For this review, take the finished solid that the model builds, in its own axes (mm). A direction names the side the tool comes from. Round coordinates to 2 decimals unless told otherwise and drop trailing zeros. Write each loop counter-clockwise with the first axis right and the second up, starting at its lowest first coordinate (ties: lowest second). Pieces come first, ordered by that corner, then holes.
from build123d import *

# Parameters (mm, degrees)
SKETCH_1_R      = 12
SKETCH_1_R_2    = 2
EXTRUDE_1_DEPTH = 3
SKETCH_1_3_R    = 2.25
EXTRUDE_2_DEPTH = 5
EXTRUDE_START   = 3
SKETCH_1_4_R    = 6
SKETCH_1_4_R_2  = 2
EXTRUDE_3_DEPTH = 3
EXTRUDE_START_2 = 6
SKETCH_1_5_R    = 6
EXTRUDE_5_DEPTH = 1
SKETCH_2_R      = 3.5
EXTRUDE_4_DEPTH = 8


with BuildPart() as part:
    # 草图1 → 凸台-拉伸1 (new body)
    with BuildSketch(Plane.XY):
        Circle(SKETCH_1_R)
        Circle(SKETCH_1_R_2, mode=Mode.SUBTRACT)
    extrude(amount=EXTRUDE_1_DEPTH)

    # 草图1<3> → 凸台-拉伸2 (add)
    with BuildSketch(Plane.XY):
        with Locations((0, 8.4)):
            Circle(SKETCH_1_3_R)
        with Locations((7.274613392, -4.2)):
            Circle(SKETCH_1_3_R)
        with Locations((-7.274613392, -4.2)):
            Circle(SKETCH_1_3_R)
    extrude(amount=-EXTRUDE_2_DEPTH)

    # 草图1<4> → 凸台-拉伸3 (add)
    with BuildSketch(Plane.XY.offset(EXTRUDE_START)):
        Circle(SKETCH_1_4_R)
        Circle(SKETCH_1_4_R_2, mode=Mode.SUBTRACT)
    extrude(amount=EXTRUDE_3_DEPTH)

    # 草图1<5> → 凸台-拉伸5 (add)
    with BuildSketch(Plane.XY.offset(EXTRUDE_START_2)):
        Circle(SKETCH_1_5_R)
    extrude(amount=EXTRUDE_5_DEPTH)

    # 草图2 → 凸台-拉伸4 (add)
    with BuildSketch(Plane.XY.offset(7)):
        Circle(SKETCH_2_R)
        Polygon((-1.204280479, -1.204280479), (-2.304280479, -1.204280479), (-2.304280479, 1.204280479), (-1.204280479, 1.204280479), (-1.204280479, 2.304280479), (1.204280479, 2.304280479), (1.204280479, 1.204280479), (2.304280479, 1.204280479), (2.304280479, -1.204280479), (1.204280479, -1.204280479), (1.204280479, -2.304280479), (-1.204280479, -2.304280479), align=None, mode=Mode.SUBTRACT)
    extrude(amount=EXTRUDE_4_DEPTH)


solid = part.part
(1) For pin 1 Ø0.6 at (x, z) = (2, 11) entering from +Y; pin 2 Ø2.5 at (y, z) = (0, 12) entering from +X; pin 3 Ø1.9 at (x, z) = (0, 11) entering from +Y, all flat-tipped, find the tip position at first contact; note any pin that passes through.
Geometry check:
pin 1: stops at y = 3.06
pin 2: stops at x = 3.5
pin 3: stops at y = 3.5
(2) For faces 4 (the face through (0, -2, 3)), 5 (the face through (0, 2.304, 11)), 6 (the face through (-7, -4, -5)), list the 3-axis set-ups (+Z, -Z, +X, -X, +Y, -Y) from which the entire face can be reached by the end or side of a thin tool; tool diameter is ignored.
Geometry check:
face 4: -Z
face 5: +Z
face 6: -Z, +X, -X, +Y, -Y
(3) For line 1 along Y through (x, z) = (0, 1.3); line 2 along Z through (x, y) = (6.75, -0.75); line 3 along Z through (x, y) = (-0.75, 1.5), list the stretches that pass through material, from the lowest coordinate up.
Geometry check:
line 1: y = -12 to -2, 2 to 12
line 2: z = 0 to 3
line 3: z = 6 to 7
(4) We need section B-B, the plane x = 0. Give the boundary of the cut face in (y, z), and give its area (3 significant figures).
Geometry check:
outline: (-12, 0) - (-2, 0) - (-2, 6) - (2, 6) - (2, 0) - (6.15, 0) - (6.15, -5) - (10.65, -5) - (10.65, 0) - (12, 0) - (12, 3) - (6, 3) - (6, 7) - (3.5, 7) - (3.5, 15) - (2.3, 15) - (2.3, 7) - (-2.3, 7) - (-2.3, 15) - (-3.5, 15) - (-3.5, 7) - (-6, 7) - (-6, 3) - (-12, 3) - close
area: 138 mm2
(5) We need section A-A, the plane z = 9.75. Give the boundary of the cut face in (x, y).
Geometry check:
outline: circle Ø7 at (0, 0); hole (-2.3, -1.2) - (-1.2, -1.2) - (-1.2, -2.3) - (1.2, -2.3) - (1.2, -1.2) - (2.3, -1.2) - (2.3, 1.2) - (1.2, 1.2) - (1.2, 2.3) - (-1.2, 2.3) - (-1.2, 1.2) - (-2.3, 1.2) - close
(6) We need section D-D, the plane z = -3.5. Give the boundary of the cut face in (x, y), and give its area (3 significant figures).
Geometry check:
outline: circle Ø4.5 at (-7.27, -4.2); circle Ø4.5 at (0, 8.4); circle Ø4.5 at (7.27, -4.2)
area: 47.7 mm2
(7) Mouldability with a two-part tool opening along X and no side actions: class faces 1 (the face through (3, -3, 7)), 2 (the face through (-11.99, 0.53, 1.48)), 3 (the face through (1.204, 2, 11)) as pulls with the +X half, pulls with the -X half, needs draft (parallel to the pull), parting line crosses it, or undercut.
Geometry check:
face 1: needs draft
face 2: parting line crosses it
face 3: undercut
(8) We need section C-C, the plane y = 0. Give the boundary of the cut face in (x, z), and give its area (3 significant figures).
Geometry check:
outline: (-12, 0) - (-2, 0) - (-2, 6) - (2, 6) - (2, 0) - (12, 0) - (12, 3) - (6, 3) - (6, 7) - (3.5, 7) - (3.5, 15) - (2.3, 15) - (2.3, 7) - (-2.3, 7) - (-2.3, 15) - (-3.5, 15) - (-3.5, 7) - (-6, 7) - (-6, 3) - (-12, 3) - close
area: 115 mm2
